```python
from build123d import *

# Parameters (mm, degrees)
F0_W     = 20
F0_H     = 50
F0_W_2   = 12
F0_H_2   = 40
F1_DEPTH = 100
F2_W     = 70
F2_H     = 40
F3_DEPTH = 25


with BuildPart() as f1:
    # F0 (on Front) → F1 (new body)
    with BuildSketch(Plane.XZ):
        with Locations((10, -25)):
            Rectangle(F0_W, F0_H)
        with Locations((10, -25)):
            Rectangle(F0_W_2, F0_H_2, mode=Mode.SUBTRACT)
    extrude(amount=F1_DEPTH)

    # F2 (on face) → F3 (cut)
    with BuildSketch(Plane.YZ.offset(20)):
        with Locations((-55, -25)):
            Rectangle(F2_W, F2_H)
    extrude(amount=-F3_DEPTH, mode=Mode.SUBTRACT)


solid = f1.part
```
Geometry check sheet. Reference: the model listing, model coordinates, mm. A direction names the side the tool comes from. Round coordinates to 2 decimals unless told otherwise and drop trailing zeros. Loops run counter-clockwise (first coordinate to the right, second up) from the corner with the lowest first, then second, coordinate; pieces in that order, holes last. Notation, with made-up numbers: M 42.25,33 L 61.25,33 A8 ccw 61.25,47 Z; hole C -31,-35.5 d11. An arc over 180 degrees is marked long. Return JSON: item names as keys, results as strings. Group by question number.
(1) Go/stop test with a flat-tipped pin: pin 1 (1.2 mm diameter, centred on x = 2.5, z = -33, fed in from +Y). Record where the tip stops, or that it passes through.
(2) Set-up check for faces 5 (the face through (18, -20, -25)), 6 (the face through (4, -95, -25)), 7 (the face through (10, -51, -5)): record each of +Z, -Z, +X, -X, +Y, -Y from which the full face is reachable in a straight line by a thin tool's end or side.
(3) Section check C-C, the plane z = -6.5. Enter the section's corners in (x, y).
(4) Section check D-D, the plane y = -13.5. Enter the section's corners in (x, z).
(5) Section check A-A, the plane y = -64.5. Enter the section's corners in (x, z).
(6) Scan lines: line 1 along Y through (x, z) = (3, -42.5); line 2 along Z through (x, y) = (6.5, -79.5); line 3 along X through (y, z) = (-3.5, -29.5). Record each from-to range of solid material in increasing order. Write a range as [from, to].
(7) Section check B-B, the plane x = 7.5. Enter the section's corners in (y, z), and give its area (3 significant figures).
(8) Mould release check, pull along Y, two halves, no side actions. Record for faces 1 (the face through (3, -100, -25)), 2 (the face through (2, -20, -25)), 3 (the face through (16, -95, -25)), 4 (the face through (2, -90, -25)): pulls with the +Y half, pulls with the -Y half, needs draft (parallel to the pull), parting line crosses it, or undercut.
Data:
{
 "1": {"pin 1": "y = 0"},
 "2": {"face 5": "+X, -X", "face 6": "+Y, -Y", "face 7": "none"},
 "3": {"outline": "M 0,-100 L 4,-100 L 4,-90 L 0,-90 Z; M 0,-20 L 4,-20 L 4,0 L 0,0 Z; M 16,-100 L 20,-100 L 20,-90 L 16,-90 Z; M 16,-20 L 20,-20 L 20,0 L 16,0 Z"},
 "4": {"outline": "M 0,-50 L 20,-50 L 20,0 L 0,0 Z; hole M 4,-45 L 16,-45 L 16,-5 L 4,-5 Z"},
 "5": {"outline": "M 0,-50 L 20,-50 L 20,-45 L 0,-45 Z; M 0,-5 L 20,-5 L 20,0 L 0,0 Z"},
 "6": {"line 1": "[-100, -90], [-20, 0]", "line 2": "[-50, -45], [-5, 0]", "line 3": "[0, 4], [16, 20]"},
 "7": {"outline": "M -100,-50 L 0,-50 L 0,-45 L -100,-45 Z; M -100,-5 L 0,-5 L 0,0 L -100,0 Z", "area": "1,000 mm²"},
 "8": {"face 1": "pulls with the -Y half", "face 2": "undercut", "face 3": "needs draft", "face 4": "undercut"}
}
